Here's the drawing with two shaded views (mm, measured from the low corner). I have some questions. A direction names the side the tool comes from. Give positions to 0.01 mm unless a question says otherwise; leave off trailing zeros. Loops run counter-clockwise (first coordinate to the right, second up) from the corner with the lowest first, then second, coordinate; pieces in that order, holes last. Notation, with made-up numbers: M 35.5,60 L 61.5,60 A12 ccw 61.5,72 Z; hole C 86.5,36 d3. An arc over 180 degrees is marked long. Answer in a Markdown table with one row per item. Add a question column.
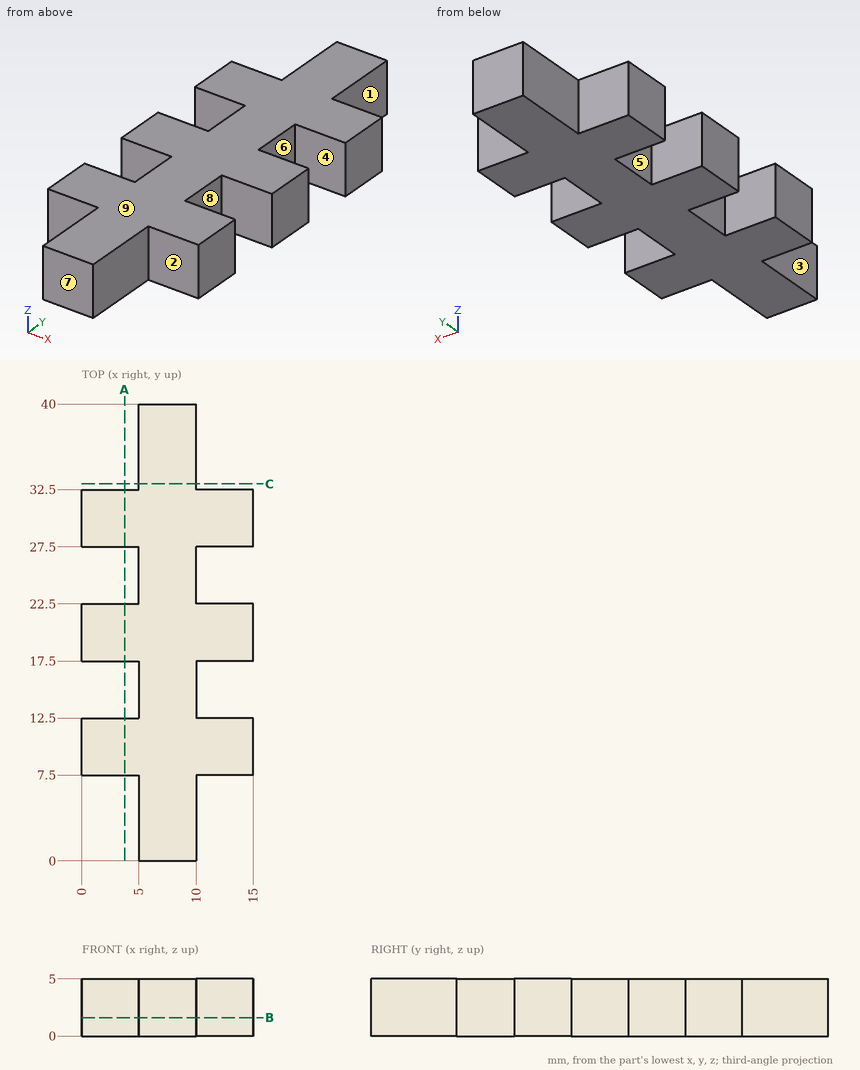
Item 1: Suppose I cut it at B-B (z = 1.6). List the corners of the cut face in (x, y) for me.
Item 2: If we mould it in two halves opening along Y, with no side actions, what happens to the marked faces 6, 7, 8 and 9? For each: +Y half, -Y half, draft (parallel to the pull), parting line (faces both ways), or undercut.
Item 3: I need wall thicknesses on L1, parallel to Y at x = 13.5, z = 4.45; L2, parallel to X at y = 38, z = 1. Which ranges of each line are inside material? Lowest first, please.
Item 4: Suppose I cut it at A-A (x = 3.75). List the corners of the cut face in (y, z) for me, then the cut area to 3 significant figures.
Item 5: For P1, Ø2.5, axis at x = 1.5, z = 2, coming from the -Y side; P2, Ø2.5, axis at y = 24, z = 2.5, coming from the -X side; P3, Ø2, axis at x = 12.5, z = 0.5, coming from the +Y side, each with a flat end and sliding along its axis, tell me the tip position at first contact or that it passes through.
Item 6: Suppose I cut it at C-C (y = 33). List the corners of the cut face in (x, z) for me.
Item 7: For the marked faces 1, 2, 3, 4 and 5, which set-ups out of +Z, -Z, +X, -X, +Y, -Y let a thin tool reach every point of the face, with its end or its side?
Values found:
| question | item | result |
|---|---|---|
| 1 | outline | M 0,7.5 L 5,7.5 L 5,0 L 10,0 L 10,7.5 L 15,7.5 L 15,12.5 L 10,12.5 L 10,17.5 L 15,17.5 L 15,22.5 L 10,22.5 L 10,27.5 L 15,27.5 L 15,32.5 L 10,32.5 L 10,40 L 5,40 L 5,32.5 L 0,32.5 L 0,27.5 L 5,27.5 L 5,22.5 L 0,22.5 L 0,17.5 L 5,17.5 L 5,12.5 L 0,12.5 Z |
| 2 | face 6 | undercut |
| 2 | face 7 | -Y half |
| 2 | face 8 | undercut |
| 2 | face 9 | draft |
| 3 | L1 | 7.5 to 12.5, 17.5 to 22.5, 27.5 to 32.5 |
| 3 | L2 | 5 to 10 |
| 4 | outline | M 7.5,0 L 12.5,0 L 12.5,5 L 7.5,5 Z; M 17.5,0 L 22.5,0 L 22.5,5 L 17.5,5 Z; M 27.5,0 L 32.5,0 L 32.5,5 L 27.5,5 Z |
| 4 | area | 75.0 mm² |
| 5 | P1 | y = 7.5 |
| 5 | P2 | x = 5 |
| 5 | P3 | y = 32.5 |
| 6 | outline | M 5,0 L 10,0 L 10,5 L 5,5 Z |
| 7 | face 1 | +Z, -Z, +X, +Y |
| 7 | face 2 | +Z, -Z, +X, -Y |
| 7 | face 3 | +Z, -Z, -X, -Y |
| 7 | face 4 | +Z, -Z, +X |
| 7 | face 5 | +Z, -Z, -X |
